Part model, mm, in its own coordinate system. Face numbers are marked on the shaded views. A direction names the side the tool comes from. Coordinates: 2 decimals unless noted, no trailing zeros. Order: outer loops, then holes, each group sorted by start corner. A loop starts at its lowest first (then second) coordinate and runs counter-clockwise, first axis right, second up. Notation, with made-up numbers: M 83,89 L 136,89 A26 cw 136,103 Z; hole C 75,71.5 d11. An arc over 180 degrees is marked long. Answer in a Markdown table with one row per item. Add a question column.
from build123d import *

# Parameters (mm, degrees)
SKETCH1_W              = 57.15
SKETCH1_H              = 177.8
BOSS_EXTRUDE1_DEPTH    = 22.225
CUT_EXTRUDE1_DEPTH     = 149.86
FILLET1_R              = 17.145
FILLET2_R              = 6.35
SKETCH4_W              = 3.81
SKETCH4_H              = 2.54
CUT_EXTRUDE2_DEPTH     = 215.392
CUT_EXTRUDE5_START     = 14.224
CUT_EXTRUDE5_DEPTH     = 14.224
SKETCH6_R              = 3.81
CUT_EXTRUDE6_DEPTH     = 117.856
SKETCH7_R              = 3.81
BOSS_EXTRUDE2_DEPTH    = 6.35
CUT_EXTRUDE7_START     = 9.525
CUT_EXTRUDE7_OUTLINE_R = 3.81
CUT_EXTRUDE7_DEPTH     = 38.1
FILLET3_R              = 6.35


# Read off the part's stored shape, not the designer's step: Cut-Extrude7
with BuildPart() as part:
    # Sketch1 → Boss-Extrude1 (new body)
    with BuildSketch(Plane.XY):
        with Locations((28.575, 88.9)):
            Rectangle(SKETCH1_W, SKETCH1_H)
    extrude(amount=BOSS_EXTRUDE1_DEPTH)

    # Sketch3 → Cut-Extrude1 (cut)
    with BuildSketch(Plane.ZY):
        Polygon((0, 0), (12.065, 177.8), (0, 177.8), align=None)
    extrude(amount=-CUT_EXTRUDE1_DEPTH, mode=Mode.SUBTRACT)

    # Fillet1
    fillet1_edges = [part.edges().sort_by_distance(p)[0] for p in [
        (0, 177.8, 17.145),
        (57.15, 177.8, 17.145),
    ]]
    fillet(fillet1_edges, radius=FILLET1_R)

    # Fillet2
    fillet2_edges = [part.edges().sort_by_distance(p)[0] for p in [
        (28.575, 0, 0),
        (28.575, 0, 22.225),
    ]]
    fillet(fillet2_edges, radius=FILLET2_R)

    # Sketch4 → Cut-Extrude2 (cut)
    with BuildSketch(Plane.XZ):
        with Locations((1.905, 20.955)):
            Rectangle(SKETCH4_W, SKETCH4_H)
        with Locations((9.525, 20.955)):
            Rectangle(SKETCH4_W, SKETCH4_H)
        with Locations((17.145, 20.955)):
            Rectangle(SKETCH4_W, SKETCH4_H)
        with Locations((24.765, 20.955)):
            Rectangle(SKETCH4_W, SKETCH4_H)
        with Locations((32.385, 20.955)):
            Rectangle(SKETCH4_W, SKETCH4_H)
        with Locations((40.005, 20.955)):
            Rectangle(SKETCH4_W, SKETCH4_H)
        with Locations((47.625, 20.955)):
            Rectangle(SKETCH4_W, SKETCH4_H)
        with Locations((55.245, 20.955)):
            Rectangle(SKETCH4_W, SKETCH4_H)
    extrude(amount=-CUT_EXTRUDE2_DEPTH, mode=Mode.SUBTRACT)

    # Sketch5 → Cut-Extrude5 (cut)
    with BuildSketch(Plane.XY.offset(19.685).offset(CUT_EXTRUDE5_START)):
        with BuildLine():
            Line((2.54, 160.655), (0, 160.655))
            ThreePointArc((0, 160.655), (0.980538982, 166.37), (3.81, 171.431307345))
            ThreePointArc((3.81, 171.431307345), (5.583362193, 173.315156248), (7.62, 174.910714644))
            ThreePointArc((7.62, 174.910714644), (9.46546693, 175.983920276), (11.43, 176.819461018))
            ThreePointArc((11.43, 176.819461018), (13.309998856, 177.365589195), (15.24, 177.693837989))
            ThreePointArc((15.24, 177.693837989), (16.191022095, 177.773438923), (17.145, 177.8))
            Line((17.145, 177.8), (19.05, 177.8))
            Line((19.05, 177.8), (22.86, 177.8))
            Line((22.86, 177.8), (26.67, 177.8))
            Line((26.67, 177.8), (30.48, 177.8))
            Line((30.48, 177.8), (34.29, 177.8))
            Line((34.29, 177.8), (38.1, 177.8))
            Line((38.1, 177.8), (40.005, 177.8))
            ThreePointArc((40.005, 177.8), (40.958977905, 177.773438923), (41.91, 177.693837989))
            ThreePointArc((41.91, 177.693837989), (43.840001144, 177.365589195), (45.72, 176.819461018))
            ThreePointArc((45.72, 176.819461018), (47.68453307, 175.983920276), (49.53, 174.910714644))
            ThreePointArc((49.53, 174.910714644), (51.566637807, 173.315156248), (53.34, 171.431307345))
            ThreePointArc((53.34, 171.431307345), (56.169461018, 166.37), (57.15, 160.655))
            Line((57.15, 160.655), (54.61, 160.655))
            ThreePointArc((54.61, 160.655), (53.774726052, 165.523333333), (51.364444444, 169.834817368))
            ThreePointArc((51.364444444, 169.834817368), (49.853802577, 171.439577544), (48.118888889, 172.798756919))
            ThreePointArc((48.118888889, 172.798756919), (46.546824467, 173.712969124), (44.873333333, 174.424726052))
            ThreePointArc((44.873333333, 174.424726052), (43.271852826, 174.889946351), (41.627777778, 175.169565694))
            ThreePointArc((41.627777778, 175.169565694), (40.817647845, 175.237373897), (40.005, 175.26))
            Line((40.005, 175.26), (38.1, 175.26))
            Line((38.1, 175.26), (34.29, 175.26))
            Line((34.29, 175.26), (30.48, 175.26))
            Line((30.48, 175.26), (26.67, 175.26))
            Line((26.67, 175.26), (22.86, 175.26))
            Line((22.86, 175.26), (19.05, 175.26))
            Line((19.05, 175.26), (17.145, 175.26))
            ThreePointArc((17.145, 175.26), (16.332352155, 175.237373897), (15.522222222, 175.169565694))
            ThreePointArc((15.522222222, 175.169565694), (13.878147174, 174.889946351), (12.276666667, 174.424726052))
            ThreePointArc((12.276666667, 174.424726052), (10.603175533, 173.712969124), (9.031111111, 172.798756919))
            ThreePointArc((9.031111111, 172.798756919), (7.296197423, 171.439577544), (5.785555556, 169.834817368))
            ThreePointArc((5.785555556, 169.834817368), (3.375273948, 165.523333333), (2.54, 160.655))
        make_face()
    extrude(amount=-CUT_EXTRUDE5_DEPTH, mode=Mode.SUBTRACT)

    # Sketch6 → Cut-Extrude6 (cut)
    with BuildSketch(Plane.ZY):
        with Locations((9.98506493, 9.525)):
            Circle(SKETCH6_R)
    extrude(amount=-CUT_EXTRUDE6_DEPTH, mode=Mode.SUBTRACT)

    # Sketch7 → Boss-Extrude2 (add)
    with BuildSketch(Plane.ZY):
        with BuildLine():
            Line((9.611876604, 141.648707852), (10.901589286, 160.655))
            Line((10.901589286, 160.655), (-9.13281329, 157.365703773))
            ThreePointArc((-9.13281329, 157.365703773), (-15.243978439, 149.813024962), (-8.444101503, 142.873934938))
            Line((-8.444101503, 142.873934938), (9.611876604, 141.648707852))
        make_face()
        with Locations((-7.949711075, 150.159680223)):
            Circle(SKETCH7_R, mode=Mode.SUBTRACT)
    boss_extrude2 = extrude(amount=-BOSS_EXTRUDE2_DEPTH)

    # Mirror1: Boss-Extrude2 across plane
    add(boss_extrude2.mirror(Plane.ZY.offset(-28.575)))

    # Cut-Extrude7 outline → Cut-Extrude7 (cut)
    with BuildSketch(Plane.YZ.offset(CUT_EXTRUDE7_START)):
        with BuildLine():
            Line((6.779904227, 0.46006493), (25.786196375, 1.749777611))
            Line((25.786196375, 1.749777611), (24.784609855, 16.51))
            Line((24.784609855, 16.51), (0.031829774, 16.51))
            ThreePointArc((0.031829774, 16.51), (0.007962436, 16.192898622), (0, 15.875))
            Line((0, 15.875), (0, 6.795495646))
            ThreePointArc((0, 6.795495646), (2.014529544, 2.155862479), (6.779904227, 0.46006493))
        make_face()
        with Locations((9.525, 9.98506493)):
            Circle(CUT_EXTRUDE7_OUTLINE_R, mode=Mode.SUBTRACT)
    extrude(amount=CUT_EXTRUDE7_DEPTH, mode=Mode.SUBTRACT)

    # Fillet3
    fillet3_edges = [part.edges().sort_by_distance(p)[0] for p in [
        (28.575, 25.786196375, 1.749777611),
        (28.575, 24.784609855, 16.51),
    ]]
    fillet(fillet3_edges, radius=FILLET3_R)


solid = part.part
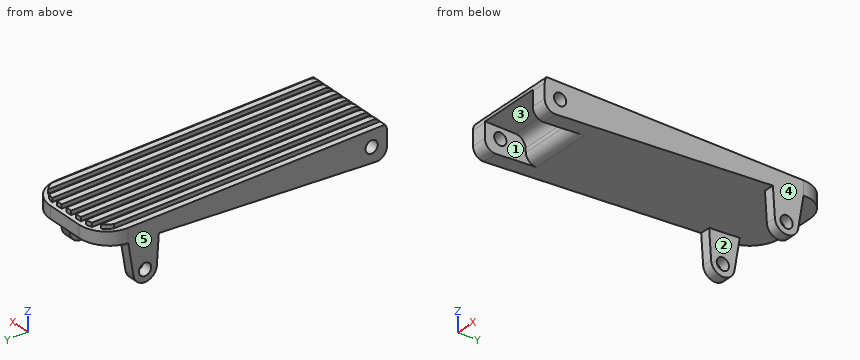
(1) Drop flat-ended pins along their axis: P1, Ø1.3, axis at x = 20.5, z = 21.5, coming from the +Y side; P2, Ø0.8, axis at y = 104, z = 21, coming from the +X side; P3, Ø4, axis at x = 48.5, z = 12, coming from the +Y side. Give the stop position or say it passes through.
(2) 3-axis set-ups, long thin cutter, end or side, ignore diameter. For the marked faces 1 and 2: which of +Z, -Z, +X, -X, +Y, -Y reach the whole face in a straight line?
(3) Slice it at A-A (z = 4.5). List the corners of the cut face in (x, y) (3 decimals).
(4) Pull direction X, two halves, no side cores. Call the marked faces 3, 4 and 5: pulls with the +X half, pulls with the -X half, needs draft (parallel to the pull), parting line crosses it, or undercut.
(5) Wall check: line 1 (X direction, y = 161, z = 12); line 2 (Z direction, x = 15.5, y = 140.5) (3 decimals); line 3 (Z direction, x = 46, y = 15) (3 decimals). Give the ranges that are in metal, low to high.
Computed:
| question | item | result |
|---|---|---|
| 1 | P1 | stops at y = 175.26 |
| 1 | P2 | stops at x = 53.34 |
| 1 | P3 | stops at y = 176.52 |
| 2 | face 1 | -Z, -Y |
| 2 | face 2 | -Z, +Y |
| 3 | outline | M 0,0.429 L 9.525,0.429 L 9.525,26.772 L 47.625,26.772 L 47.625,0.429 L 57.15,0.429 L 57.15,66.316 L 0,66.316 Z; M 0,141.996 L 6.35,141.996 L 6.35,159.604 L 0,159.604 Z; M 50.8,141.996 L 57.15,141.996 L 57.15,159.604 L 50.8,159.604 Z |
| 4 | face 3 | undercut |
| 4 | face 4 | pulls with the +X half |
| 4 | face 5 | pulls with the -X half |
| 5 | line 1 | x = 0 to 57.15 |
| 5 | line 2 | z = 9.534 to 19.685 |
| 5 | line 3 | z = 16.51 to 19.685 |
